Source: CAD feature listing. Evaluate the final solid. Frame: model axes, mm. A direction names the side the tool comes from. Give positions to 0.01 mm unless a question says otherwise; leave off trailing zeros. Order: outer loops, then holes, each group sorted by start corner. A loop starts at its lowest first (then second) coordinate and runs counter-clockwise, first axis right, second up. Notation, with made-up numbers: M -15,25.5 L 26,25.5 A30 cw 26,59.5 Z; hole C -8,10.25 d10. An arc over 180 degrees is marked long. Answer as a JSON object with one key per item and string values. Group by question number.
1. Pull-direction query (X, two-part tool) for faces 1 (the flat face through (-60, 2, 0)), 2 (the flat face through (-1, 0, 9)), 3 (the flat face through (-22.054, 0, -1)); classes: +X half, -X half, draft (parallel to the pull), parting line (faces both ways), or undercut.
2. Material intervals for L1, parallel to Z at x = -48, y = -6.8; L2, parallel to Z at x = -22, y = 7.5; L3, parallel to Y at x = -49, z = -3.5, sorted ascending. Write a range as [from, to].
3. Section query D-D (x = -48). Output: boundary loops of the cut face in (y, z).
4. Section query B-B (z = 0). Output: boundary loops of the cut face in (x, y).
5. Set-up query: faces 4 (the cylindrical face through (-53, -7, 0)), 5 (the flat face through (-1, 0, -9)), 6 (the flat face through (0, 0, -6)). Return all of +Z, -Z, +X, -X, +Y, -Y with unobstructed straight access to the full face (end or side cutting, diameter ignored); none if empty.
6. Section query C-C (x = 12.5). Output: boundary loops of the cut face in (y, z), plus the area to 3 significant figures.
7. Section query A-A (y = 4.5). Output: boundary loops of the cut face in (x, z).
8. Pin query (flat end, axial travel): P1, Ø3, axis at x = -48, z = 0, coming from the +Y side; P2, Ø3, axis at x = -46.5, z = 0.5, coming from the -Y side. Return the tip coordinate at first contact, or that it passes through.
from build123d import *

# Parameters (mm, degrees)
F0_W           = 120
F0_H           = 18
F1_DEPTH       = 9
F2_W           = 44.108732
F2_H           = 10
F3_DEPTH       = 25
F5_D           = 5
F5_CBORE_D     = 10
F5_CBORE_DEPTH = 5
F6_SIZE        = 5


with BuildPart() as f1:
    # F0 (on Top) → F1 (new body, symmetric)
    with BuildSketch(Plane.XY):
        Rectangle(F0_W, F0_H)
    extrude(amount=F1_DEPTH, both=True)

    # F2 (on face) → F3 (cut)
    with BuildSketch(Plane.XZ.offset(9)):
        with Locations((0, -1)):
            Rectangle(F2_W, F2_H)
    extrude(amount=-F3_DEPTH, mode=Mode.SUBTRACT)

    # F5 (through all)
    with Locations(Plane.XZ.offset(9)):
        with Locations((-48, 0)):
            CounterBoreHole(F5_D / 2, F5_CBORE_D / 2, F5_CBORE_DEPTH)

    # F6
    f6_edges = [f1.edges().sort_by_distance(p)[0] for p in [
        (60, -9, 0),
        (-60, -9, 0),
    ]]
    chamfer(f6_edges, length=F6_SIZE)


solid = f1.part
Answer sheet:
{
 "1": {"face 1": "-X half", "face 2": "draft", "face 3": "undercut"},
 "2": {"L1": "[-9, -5], [5, 9]", "L2": "[-9, -6], [4, 9]", "L3": "[-4, 9]"},
 "3": {"outline": "M -9,-9 L 9,-9 L 9,-2.5 L -4,-2.5 L -4,-5 L -9,-5 Z; M -9,5 L -4,5 L -4,2.5 L 9,2.5 L 9,9 L -9,9 Z"},
 "4": {"outline": "M -60,-4 L -55,-9 L -53,-9 L -53,-4 L -50.5,-4 L -50.5,9 L -60,9 Z; M -45.5,-4 L -43,-4 L -43,-9 L -22.05,-9 L -22.05,9 L -45.5,9 Z; M 22.05,-9 L 55,-9 L 60,-4 L 60,9 L 22.05,9 Z"},
 "5": {"face 4": "-Y", "face 5": "-Z, +X, -X, +Y, -Y", "face 6": "+Y, -Y"},
 "6": {"outline": "M -9,-9 L 9,-9 L 9,-6 L -9,-6 Z; M -9,4 L 9,4 L 9,9 L -9,9 Z", "area": "144 mm^2"},
 "7": {"outline": "M -60,-9 L 60,-9 L 60,9 L -60,9 Z; hole C -48,0 d5; hole M -22.05,-6 L 22.05,-6 L 22.05,4 L -22.05,4 Z"},
 "8": {"P1": "through", "P2": "y = -4"}
}
